The model under review builds one solid part; all positions refer to its coordinate system, in mm. Face numbers are marked on the shaded views. Round coordinates to 2 decimals unless told otherwise and drop trailing zeros. Order: outer loops, then holes, each group sorted by start corner. A loop starts at its lowest first (then second) coordinate and runs counter-clockwise, first axis right, second up. Notation, with made-up numbers: (27, -39) -> (86, -39) arc R11 ccw to (86, -22) -> close; hole circle Ø11 at (74, 66.25). An arc over 180 degrees is marked (long way). Return JSON: item names as keys, results as strings. Group by question number.
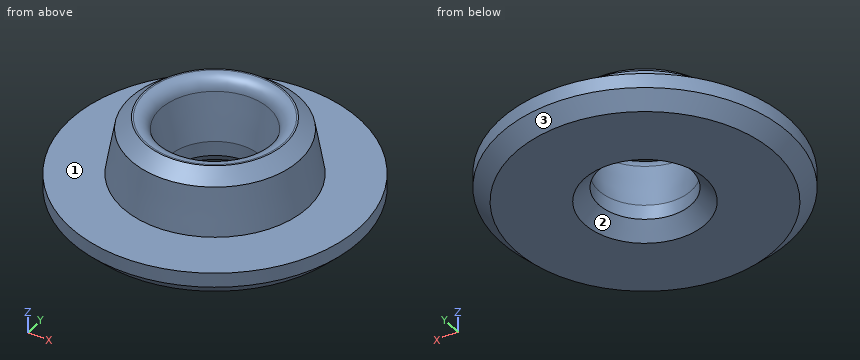
from build123d import *

# Parameters (mm, degrees)
F0_R     = 5
F0_R_2   = 1.6
F1_DEPTH = 1
F2_R     = 3.2
F2_R_2   = 1.6
F3_DEPTH = 2
F3_TAPER = 10
F5_R     = 0.5


# Not quite as in the source:
# - a fillet or chamfer that OpenCascade refuses, or shapes differently, is made with other operations: its cross-section is extruded or revolved along the edge and cut away or added


with BuildPart() as f1:
    # F0 (on Top) → F1 (new body)
    with BuildSketch(Plane.XY):
        Circle(F0_R)
        Circle(F0_R_2, mode=Mode.SUBTRACT)
    extrude(amount=F1_DEPTH)

    # F2 (on face) → F3 (join)
    with BuildSketch(Plane.XY.offset(1)):
        Circle(F2_R)
        Circle(F2_R_2, mode=Mode.SUBTRACT)
    extrude(amount=F3_DEPTH, taper=F3_TAPER)

    # F4: chamfer of 0.5 on 3 edges, made by hand

    # F4_s1 → F4_t2 (revolve, cut)
    with BuildSketch(Plane.XZ):
        Polygon((5, 0.5), (4.5, 0), (5, 0), align=None)
    revolve(axis=Axis((0, 0, 0), (0, 0, 1)), mode=Mode.SUBTRACT)

    # F4_s3 → F4_t4 (revolve, cut)
    with BuildSketch(Plane.XZ):
        Polygon((2.9202000995, 2.5868240888), (2.427796223, 3), (2.8473460386, 3), align=None)
    revolve(axis=Axis((0, 0, 3), (0, 0, -1)), mode=Mode.SUBTRACT)

    # F4_s5 → F4_t6 (revolve, cut)
    with BuildSketch(Plane.XZ):
        Polygon((2.1, 0), (1.6, 0.5), (1.6, 0), align=None)
    revolve(axis=Axis((0, 0, 0), (0, 0, 1)), mode=Mode.SUBTRACT)

    # F5
    f5_edges = [f1.edges().sort_by_distance(p)[0] for p in [
        (-1.952654, 0, 3),
    ]]
    fillet(f5_edges, radius=F5_R)


solid = f1.part
Item 1: Consider section B-B on z = 0.85. State the section outline as (x, y) points.
Item 2: Insertion check: pin 1 Ø1 at (y, z) = (0, 2.5) entering from +X. The pin has a flat end and moves straight along its axis. Give the tip position at first contact, or say it passes through.
Item 3: Wall thickness on line 1 along Y through (x, z) = (0, 0.6); line 2 along Y through (x, z) = (-1.5, 1.75); line 3 along Z through (x, y) = (-3.25, -2.5): over which ranges is each line inside the solid? List them lowest first.
Item 4: Consider section C-C on z = 2.1. State the section outline as (x, y) points, plus the area to 3 significant figures.
Item 5: Consider section A-A on x = 0. State the section outline as (y, z) points.
Item 6: The part is to be moulded in two halves that separate along X. For the marked faces 1, 2 and 3, say which applies: +X half, -X half, draft (parallel to the pull), parting line (faces both ways), or undercut.
Values:
{
 "1": {"outline": "circle Ø10 at (0, 0); hole circle Ø3.2 at (0, 0)"},
 "2": {"pin 1": "x = 3.02"},
 "3": {"line 1": "-5 to -1.6, 1.6 to 5", "line 2": "-2.68 to -0.87, 0.87 to 2.68", "line 3": "0 to 1"},
 "4": {"outline": "circle Ø6.01 at (0, 0); hole circle Ø3.59 at (0, 0)", "area": "18.3 mm^2"},
 "5": {"outline": "(-5, 0.5) -> (-4.5, 0) -> (-2.1, 0) -> (-1.6, 0.5) -> (-1.6, 1) -> (-1.88, 2.59) arc R0.5 ccw to (-2.37, 3) -> (-2.43, 3) -> (-2.92, 2.59) -> (-3.2, 1) -> (-5, 1) -> close; (1.6, 0.5) -> (2.1, 0) -> (4.5, 0) -> (5, 0.5) -> (5, 1) -> (3.2, 1) -> (2.92, 2.59) -> (2.43, 3) -> (2.37, 3) arc R0.5 ccw to (1.88, 2.59) -> (1.6, 1) -> close"},
 "6": {"face 1": "draft", "face 2": "undercut", "face 3": "parting line"}
}
